The listing builds one solid part. Answer for the finished solid, in the listing's coordinates (mm). Face numbers are marked on the shaded views. A direction names the side the tool comes from. Give positions to 0.01 mm unless a question says otherwise; leave off trailing zeros. Loops run counter-clockwise (first coordinate to the right, second up) from the corner with the lowest first, then second, coordinate; pieces in that order, holes last. Notation, with made-up numbers: M -33,18 L 25,18 A13 ccw 25,22 Z; hole C -38,86 d8. An arc over 180 degrees is marked long. One line per item, written item: value. Start each with the question number.
Q1. A cutting plane is placed at C-C, the plane x = 6.5. Determine the outline of the cut face in (y, z), and give its area (3 significant figures).
Q2. For the marked faces 1 and 2, determine the directions among +Z, -Z, +X, -X, +Y, -Y from which every point of the face is accessible in a straight line to the end or side of a thin tool.
Q3. Consider L1, parallel to Y at x = 0, z = -4.25; L2, parallel to Y at x = -1.5, z = -4.5; L3, parallel to Z at x = 4, y = -72. Determine where each line is inside the solid, lowest interval first.
Q4. A cutting plane is placed at D-D, the plane y = -75. Determine the outline of the cut face in (x, z).
Q5. A cutting plane is placed at B-B, the plane z = -6.5. Determine the outline of the cut face in (x, y), and give its area (3 significant figures).
Q6. Flat-ended cylindrical pins translate along their axes: pin 1 (2.5 mm diameter, centred on x = 1, y = -82.5, fed in from -Z); pin 2 (4 mm diameter, centred on x = 7.5, z = -6.5, fed in from -Y). Find the tip coordinate at first contact, or state that the pin passes through.
Q7. A cutting plane is placed at A-A, the plane y = -82. Determine the outline of the cut face in (x, z).
Q8. The mould has two halves that part along X. Classify the marked faces 3, 4 and 5: +X half, -X half, draft (parallel to the pull), parting line (faces both ways), or undercut.
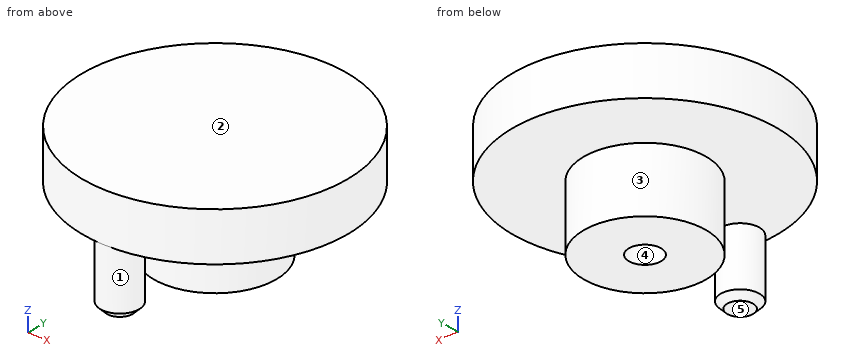
Autodesk Inventor part; units mm, degrees
ref_plane "Work Plane2" through (-3.7976, -85.7976, 4.5) normal (0, 0, 1) x (1, 0, 0)
ref_plane "YZ Plane" through (0, 0, 0) normal (1, 0, 0) x (0, 1, 0)
ref_plane "XZ Plane" through (0, 0, 0) normal (0, 1, 0) x (-1, 0, 0)
ref_plane "Work Plane1" through (0, 0, 0) normal (0, 0, 1) x (1, 0, 0)
sketch "Sketch1" plane through (0, 0, 0) normal (0, 0, 1) x (1, 0, 0)
  circle A0 centre (0, -82) radius 2.5
  circle A1 centre (0, -82) radius 11.5 construction
  circle A2 centre (0, -82) radius 9.5
  circle A3 centre (0, -99.5) radius 3
  point P0 (0, 0)
  dimension "d0" = 2
  dimension "d5" = 6
extrude "Extrusion1" add sketch "Sketch1" against normal blind 10
sketch "Sketch2" plane through (0, -82, 0) normal (0, 0, 1) x (1, 0, 0)
  circle A0 centre (0, 0) radius 17.5 construction
  circle A1 centre (0, 0) radius 20.5
  point P0 (0, 82)
  point P1 (0, -17.5)
  dimension "d6" = 3
extrude "Extrusion2" add sketch "Sketch2" along normal blind 3
chamfer "Chamfer1" distance 1 angle 45 1 edges at (-3, -99.5, -10)
sketch "Sketch3" plane through (0, -82, 3) normal (0, 0, 1) x (1, 0, 0)
  circle A0 centre (0, 0) radius 20.5
  circle A1 centre (0, 0) radius 2.5
  point P0 (0, 82)
ref_plane "Work Plane2" through (-3.7976, -85.7976, 4.5) normal (0, 0, 1) x (1, 0, 0)
extrude "Extrusion3" add sketch "Sketch3" along normal up to surface (1.5 mm away)
sketch "Sketch4" plane through (0, -82, 4.5) normal (0, 0, 1) x (1, 0, 0)
  circle A0 centre (0, 0) radius 20.5
  point P0 (0, 82)
extrude "Extrusion4" add sketch "Sketch4" along normal blind 3
properties part number "Cup_Dispenser_Transmission"
Answer block:
1. outline: M -101.44,0 L -88.93,0 L -88.93,-10 L -75.07,-10 L -75.07,0 L -62.56,0 L -62.56,7.5 L -101.44,7.5 Z
1. area: 430 mm^2
2. face 1: -Z
2. face 2: +Z, +X, -X, +Y, -Y
3. L1: -102.5 to -96.5, -91.5 to -84.5, -79.5 to -72.5
3. L2: -102.1 to -96.9, -91.38 to -84, -80 to -72.62
3. L3: 0 to 7.5
4. outline: M -19.27,0 L -6.42,0 L -6.42,-10 L 6.42,-10 L 6.42,0 L 19.27,0 L 19.27,7.5 L -19.27,7.5 Z
5. outline: C 0,-82 d19; C 0,-99.5 d6; hole C 0,-82 d5
5. area: 292 mm^2
6. pin 1: z = 0
6. pin 2: y = -89.75
7. outline: M -20.5,0 L -9.5,0 L -9.5,-10 L -2.5,-10 L -2.5,0 L 2.5,0 L 2.5,-10 L 9.5,-10 L 9.5,0 L 20.5,0 L 20.5,7.5 L -20.5,7.5 Z; hole M -2.5,3 L 2.5,3 L 2.5,4.5 L -2.5,4.5 Z
8. face 3: parting line
8. face 4: undercut
8. face 5: draft
